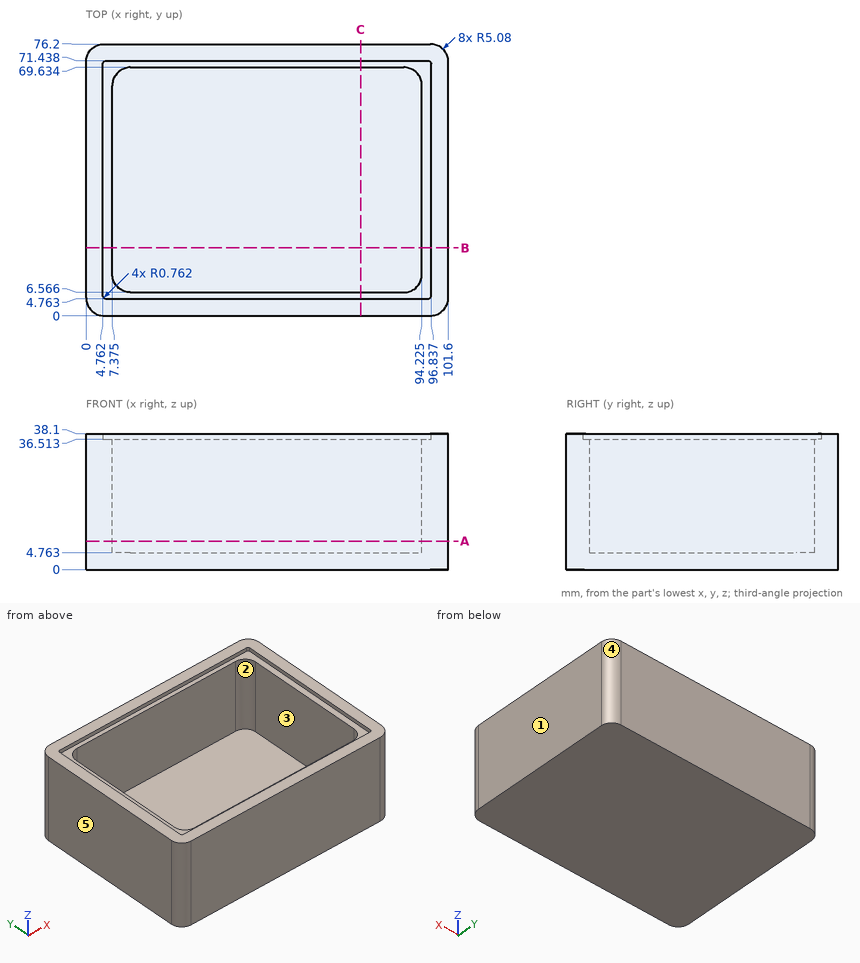
Answer from the drawing. Dimensions are ordinates in mm from the lowest x, y and z of the part. A direction names the side the tool comes from. Coordinates: 2 decimals unless noted, no trailing zeros. Loops run counter-clockwise (first coordinate to the right, second up) from the corner with the lowest first, then second, coordinate; pieces in that order, holes last.
1) Flat-ended cylindrical pins translate along their axes: pin 1 (20 mm diameter, centred on x = 68.5, y = 46.5, fed in from +Z); pin 2 (10 mm diameter, centred on x = 12, y = 57.5, fed in from +Z). Find the tip coordinate at first contact, or state that the pin passes through.
Results:
pin 1: stops at z = 4.76
pin 2: stops at z = 36.51
2) Section C-C (x = 77) is taken. Give the vertices of the cut face in (y, z), plus the area to 3 significant figures.
Results:
outline: (0, 0) - (76.2, 0) - (76.2, 38.1) - (71.44, 38.1) - (71.44, 36.51) - (69.63, 36.51) - (69.63, 4.76) - (6.57, 4.76) - (6.57, 36.51) - (4.76, 36.51) - (4.76, 38.1) - (0, 38.1) - close
area: 795 mm2
3) Consider probe 1 along X at (y, z) = (38.5, 6) (1 decimal); probe 2 along Y at (x, z) = (62.5, 31.5); probe 3 along Z at (x, y) = (47.5, 32.5). Determine where each line is inside the solid, lowest interval first.
Results:
probe 1: x = 0 to 7.4, 94.2 to 101.6
probe 2: y = 0 to 6.57, 69.63 to 76.2
probe 3: z = 0 to 4.76
4) Section A-A (z = 8) is taken. Give the vertices of the cut face in (x, y) (1 decimal).
Results:
outline: (0, 5.1) arc R5.1 ccw to (5.1, 0) - (96.5, 0) arc R5.1 ccw to (101.6, 5.1) - (101.6, 71.1) arc R5.1 ccw to (96.5, 76.2) - (5.1, 76.2) arc R5.1 ccw to (0, 71.1) - close; hole (7.4, 11.6) arc R5.1 ccw to (12.5, 6.6) - (89.1, 6.6) arc R5.1 ccw to (94.2, 11.6) - (94.2, 64.6) arc R5.1 ccw to (89.1, 69.6) - (12.5, 69.6) arc R5.1 ccw to (7.4, 64.6) - close
5) For a pull along X with two mould halves and no side action, classify the marked faces 3, 4 and 5 as +X half, -X half, draft (parallel to the pull), parting line (faces both ways), or undercut.
Results:
face 3: undercut
face 4: +X half
face 5: -X half
6) Section B-B (y = 19) is taken. Give the vertices of the cut face in (x, z) (1 decimal).
Results:
outline: (0, 0) - (101.6, 0) - (101.6, 38.1) - (96.8, 38.1) - (96.8, 36.5) - (94.2, 36.5) - (94.2, 4.8) - (7.4, 4.8) - (7.4, 36.5) - (4.8, 36.5) - (4.8, 38.1) - (0, 38.1) - close
7) For the marked faces 1 and 2, determine the directions among +Z, -Z, +X, -X, +Y, -Y from which every point of the face is accessible in a straight line to the end or side of a thin tool.
Results:
face 1: +Z, -Z, +X, +Y, -Y
face 2: +Z
